The model under review builds one solid part; all positions refer to its coordinate system, in mm. Face numbers are marked on the shaded views. A direction names the side the tool comes from. Round coordinates to 2 decimals unless told otherwise and drop trailing zeros. Order: outer loops, then holes, each group sorted by start corner. A loop starts at its lowest first (then second) coordinate and runs counter-clockwise, first axis right, second up.
Autodesk Inventor part; units mm, degrees
ref_plane "YZ Plane" through (0, 0, 0) normal (1, 0, 0) x (0, 1, 0)
ref_plane "XZ Plane" through (0, 0, 0) normal (0, 1, 0) x (-1, 0, 0)
ref_plane "XY Plane" through (0, 0, 0) normal (0, 0, 1) x (1, 0, 0)
sketch "スケッチ1" plane through (0, 0, 0) normal (0, 1, 0) x (-1, 0, 0)
  circle A0 centre (0, 0) radius 10
  line L0 (0, 10) -> (-10, 10)
  line L1 (-10, 10) -> (-10, -10)
  line L2 (-10, -10) -> (10, -10)
  line L3 (10, -10) -> (10, 0)
  dimension "d0" = 20
  dimension "d1" = 10
  dimension "d2" = 10
extrude "押し出し1" add sketch "スケッチ1" along normal mid plane 77
sketch "スケッチ2" plane through (0, -38.5, 10) normal (0, 0, 1) x (1, 0, 0)
  line L0 (10, 0) -> (10, 77)
  line L1 (0, 77) -> (10, 77)
  line L2 (0, 0) -> (0, 77)
  line L3 (10, 0) -> (0, 0)
extrude "押し出し2" cut sketch "スケッチ2" against normal blind 1
sketch "スケッチ3" plane through (-10, -38.5, -10) normal (-1, 0, 0) x (0, 0, 1)
  line L0 (0, 77) -> (10, 77)
  line L1 (10, 0) -> (10, 77)
  line L2 (10, 0) -> (0, 0)
  line L3 (0, 0) -> (0, 77)
  point P0 (10, 38.5)
extrude "押し出し3" cut sketch "スケッチ3" against normal blind 1
sketch "スケッチ4" plane through (0, -38.5, 9) normal (0, 0, 1) x (1, 0, 0)
  line L0 (0, 77) -> (10, 77)
  line L1 (10, 77) -> (10, 0)
  line L2 (10, 0) -> (0, 0)
  point P0 (0, 38.5)
  point P1 (5, 72)
  point P2 (5, 5)
  dimension "d9" = 5
  dimension "d10" = 5
  dimension "d11" = 5
hole "穴1" at (5, 33.5, 9) at (5, -33.5, 9) direction (0, 0, -1) diameter 5 depth 6
sketch "スケッチ5" plane through (0, -38.5, 0) normal (0, 1, 0) x (1, 0, 0)
  point P0 (0, 0)
hole "穴2" at (0, -38.5, 0) direction (0, 1, 0) diameter 5 depth 6
sketch "スケッチ6" plane through (-9, -38.5, -10) normal (-1, 0, 0) x (0, 0, 1)
  line L0 (0, 0) -> (0, 77)
  line L1 (0, 77) -> (10, 77)
  line L2 (10, 0) -> (0, 0)
  point P0 (10, 38.5)
  point P1 (5, 72)
  point P2 (5, 5)
  dimension "d26" = 5
  dimension "d27" = 5
  dimension "d28" = 5
  dimension "d29" = 5
hole "穴3" at (-9, 33.5, -5) at (-9, -33.5, -5) direction (1, 0, 0) diameter 5 depth 6
mirror "ミラー1" about plane through (0, 0, 0) normal (0, 1, 0) of "穴2"
sketch "スケッチ9" plane through (10, -38.5, -10) normal (1, 0, 0) x (0, 0, -1)
  line L0 (0, 77) -> (-10, 77)
  line L1 (-19, 77) -> (-19, 0)
  line L2 (0, 77) -> (-19, 77)
  line L3 (-19, 77) -> (-19, 62)
  line L4 (-19, 62) -> (0, 62)
  line L5 (0, 62) -> (0, 77)
  point P0 (-10, 38.5)
  dimension "d47" = 15
extrude "押し出し6" add sketch "スケッチ9" along normal blind 20
sketch "スケッチ10" plane through (0, 38.5, 0) normal (0, 1, 0) x (1, 0, 0)
  line L0 (30, 10) -> (30, -9)
  point P0 (0, 0)
  point P1 (20, 0)
  dimension "d50" = 10
hole "穴4" at (20, 38.5, 0) direction (0, -1, 0) diameter 6 depth 6
chamfer "面取り2" distance 3 angle 45 1 edges at (20, 38.5, -3)
chamfer "面取り3" distance 20 angle 45 1 edges at (10, 23.5, -0.5)
properties part number "base8" material "ABS プラスチック"
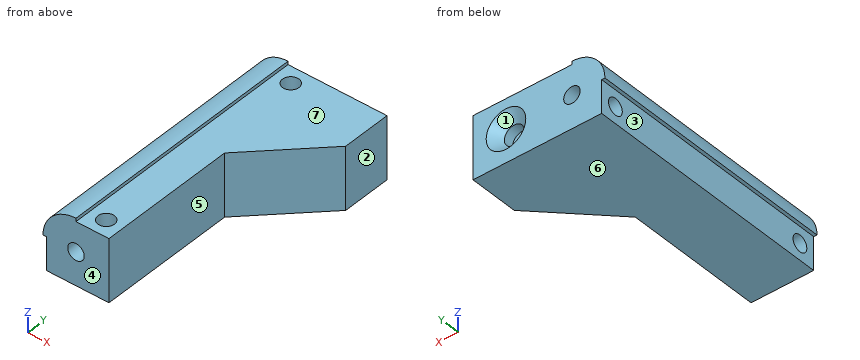
(1) Clearance check with flat-ended pins moving along their axes: P1, Ø1.5, axis at x = 0.5, z = 1, coming from the +Y side; P2, Ø11, axis at y = 15, z = -6.5, coming from the -X side; P3, Ø1.5, axis at y = 0.5, z = -1.5, coming from the +X side. State where each tip first meets the part, or that it passes through.
(2) Tool access review of the marked faces 5, 6 and 7: name each direction out of +Z, -Z, +X, -X, +Y, -Y from which nothing blocks a thin tool from reaching the whole face with its end or side.
(3) The part is to be moulded in two halves that separate along X. For the marked faces 1, 2, 3 and 4, say which applies: pulls with the +X half, pulls with the -X half, needs draft (parallel to the pull), parting line crosses it, or undercut.
(4) We need section D-D (y = -33.5). Give the boundary of the cut face in (x, z), and give its area (3 significant figures).
(5) We need section A-A (z = 8). Count the separate pieces of the cut face and the enclosed holes in it, and give its area (3 significant figures).
(6) We need section C-C (y = 1). Give the boundary of the cut face in (x, z), and give its area (3 significant figures).
(7) We need section B-B (y = 33.5). Give the boundary of the cut face in (x, z), and give its area (3 significant figures).
(8) To check wall thickness, follow L1, parallel to Y at x = -5.5, z = -6; L2, parallel to Y at x = 4.5, z = 7.5; L3, parallel to Z at x = 5, y = -16. State the ranges of each line that lie inside material, in increasing order.
Verdict:
1. P1: stops at y = 32.5
1. P2: stops at x = -9
1. P3: stops at x = 10
2. face 5: +Z, -Z, +X, -Y
2. face 6: -Z, +X, -X, +Y, -Y
2. face 7: +Z, +X, +Y, -Y
3. face 1: undercut
3. face 2: pulls with the +X half
3. face 3: pulls with the -X half
3. face 4: needs draft
4. outline: (-10, 0) - (-9, 0) - (-9, -2.5) - (-3, -2.5) - (-3, -7.5) - (-9, -7.5) - (-9, -10) - (10, -10) - (10, 9) - (7.5, 9) - (7.5, 3) - (2.5, 3) - (2.5, 9) - (0, 9) - (0, 10) arc R10 ccw to start; hole circle Ø5 at (0, 0)
4. area: 279 mm2
5. separate pieces: 1
5. enclosed holes: 2
5. area: 1,690 mm2
6. outline: (-10, 0) - (-9, 0) - (-9, -10) - (10, -10) - (10, 9) - (0, 9) - (0, 10) arc R10 ccw to start
6. area: 359 mm2
7. outline: (-10, 0) - (-9, 0) - (-9, -2.5) - (-3, -2.5) - (-3, -7.5) - (-9, -7.5) - (-9, -10) - (30, -10) - (30, 9) - (7.5, 9) - (7.5, 3) - (2.5, 3) - (2.5, 9) - (0, 9) - (0, 10) arc R10 ccw to start; hole circle Ø5 at (0, 0); hole circle Ø6 at (20, 0)
7. area: 631 mm2
8. L1: y = -38.5 to -35.79, -31.21 to 31.21, 35.79 to 38.5
8. L2: y = -38.5 to -35.95, -31.05 to 31.05, 35.95 to 38.5
8. L3: z = -10 to 9
